Build history of the part. All positions in model axes, mm. A direction names the side the tool comes from. Give positions to 0.01 mm unless a question says otherwise; leave off trailing zeros. Loops run counter-clockwise (first coordinate to the right, second up) from the corner with the lowest first, then second, coordinate; pieces in that order, holes last.
1) Flat gauge pins, fed straight in: P1, Ø8, axis at y = -107.5, z = 19.5, coming from the -X side; P2, Ø3, axis at y = -176, z = 10.5, coming from the +X side. Where does each tip first touch, or does it go through?
2) Band-saw the part on B-B on x = 1.5. List the corners of the cut face in (y, z).
3) Wall check: line 1 (Y direction, x = 11.5, z = 15.25); line 2 (Z direction, x = -5, y = -160.5); line 3 (X direction, y = 72, z = 4). Give the ranges that are in metal, low to high.
4) Band-saw the part on C-C on y = -67. List the corners of the cut face in (x, z), then the cut area to 3 significant figures.
5) Band-saw the part on A-A on z = 15. List the corners of the cut face in (x, y).
6) Two-plate mould, pull along X, no slides. Class faces 1 (the flat face through (0, 3, 3)), 2 (the flat face through (-11, -225, 14)), 3 (the flat face through (-13, 3, 15)), 4 (the flat face through (10, 3, 15)): +X half, -X half, draft (parallel to the pull), parting line (faces both ways), or undercut.
7) 3-axis set-ups, long thin cutter, end or side, ignore diameter. For faces 5 (the flat face through (13, 3, 15)), 6 (the flat face through (0, 3, 0)), 7 (the flat face through (-10, 3, 15)): which of +Z, -Z, +X, -X, +Y, -Y reach the whole face in a straight line?
```python
from build123d import *

# Parameters (mm, degrees)
SKETCH_1_W          = 30
SKETCH_1_H          = 450
EXTRUDE_1_DEPTH     = 30
SKETCH_2_W          = 2
SKETCH_2_H          = 26
CUT_EXTRUDE_1_DEPTH = 452.248268695
SHELL_1_T           = -3
CUT_EXTRUDE_2_DEPTH = 229.7116088


with BuildPart() as part:
    # 草图1 → 凸台-拉伸1 (new body)
    with BuildSketch(Plane.XY):
        Rectangle(SKETCH_1_W, SKETCH_1_H)
    extrude(amount=EXTRUDE_1_DEPTH)

    # 草图2 → 切除-拉伸1 (cut, through all)
    with BuildSketch(Plane(origin=(0, 225, 0), x_dir=(1, 0, 0), z_dir=(0, 1, 0))):
        with Locations((-14, -15)):
            Rectangle(SKETCH_2_W, SKETCH_2_H)
        with Locations((14, -15)):
            Rectangle(SKETCH_2_W, SKETCH_2_H)
    extrude(amount=-CUT_EXTRUDE_1_DEPTH, mode=Mode.SUBTRACT)

    # 抽壳1
    shell_1_openings = [part.faces().sort_by_distance(p)[0] for p in [
        (0, 225, 15),
        (0, -225, 15),
    ]]
    offset(amount=SHELL_1_T, openings=shell_1_openings)

    # 草图3 → 切除-拉伸2 (cut, through all)
    with BuildSketch(Plane(origin=(13, 0, 0), x_dir=(0, 0, -1), z_dir=(1, 0, 0))):
        with BuildLine():
            Line((-20, 205), (-10, 205))
            ThreePointArc((-10, 205), (-15, 210), (-20, 205))
        make_face()
        with BuildLine():
            Line((-20, -195), (-10, -195))
            ThreePointArc((-10, -195), (-15, -200), (-20, -195))
        make_face()
    extrude(amount=-CUT_EXTRUDE_2_DEPTH, mode=Mode.SUBTRACT)


solid = part.part
```
Findings below:
1. P1: stops at x = -13
1. P2: stops at x = 13
2. outline: (-225, 0) - (225, 0) - (225, 3) - (-225, 3) - close; (-225, 27) - (225, 27) - (225, 30) - (-225, 30) - close
3. line 1: y = -225 to -199.99, -195 to 205, 209.99 to 225
3. line 2: z = 0 to 3, 27 to 30
3. line 3: x = -13 to -10, 10 to 13
4. outline: (-15, 0) - (15, 0) - (15, 2) - (13, 2) - (13, 28) - (15, 28) - (15, 30) - (-15, 30) - (-15, 28) - (-13, 28) - (-13, 2) - (-15, 2) - close; hole (-10, 3) - (10, 3) - (10, 27) - (-10, 27) - close
4. area: 316 mm2
5. outline: (-13, -225) - (-10, -225) - (-10, -200) - (-13, -200) - close; (-13, -195) - (-10, -195) - (-10, 205) - (-13, 205) - close; (-13, 210) - (-10, 210) - (-10, 225) - (-13, 225) - close; (10, -225) - (13, -225) - (13, -200) - (10, -200) - close; (10, -195) - (13, -195) - (13, 205) - (10, 205) - close; (10, 210) - (13, 210) - (13, 225) - (10, 225) - close
6. face 1: undercut
6. face 2: draft
6. face 3: -X half
6. face 4: undercut
7. face 5: +X, +Y, -Y
7. face 6: -Z, +X, -X, +Y, -Y
7. face 7: +Y, -Y
